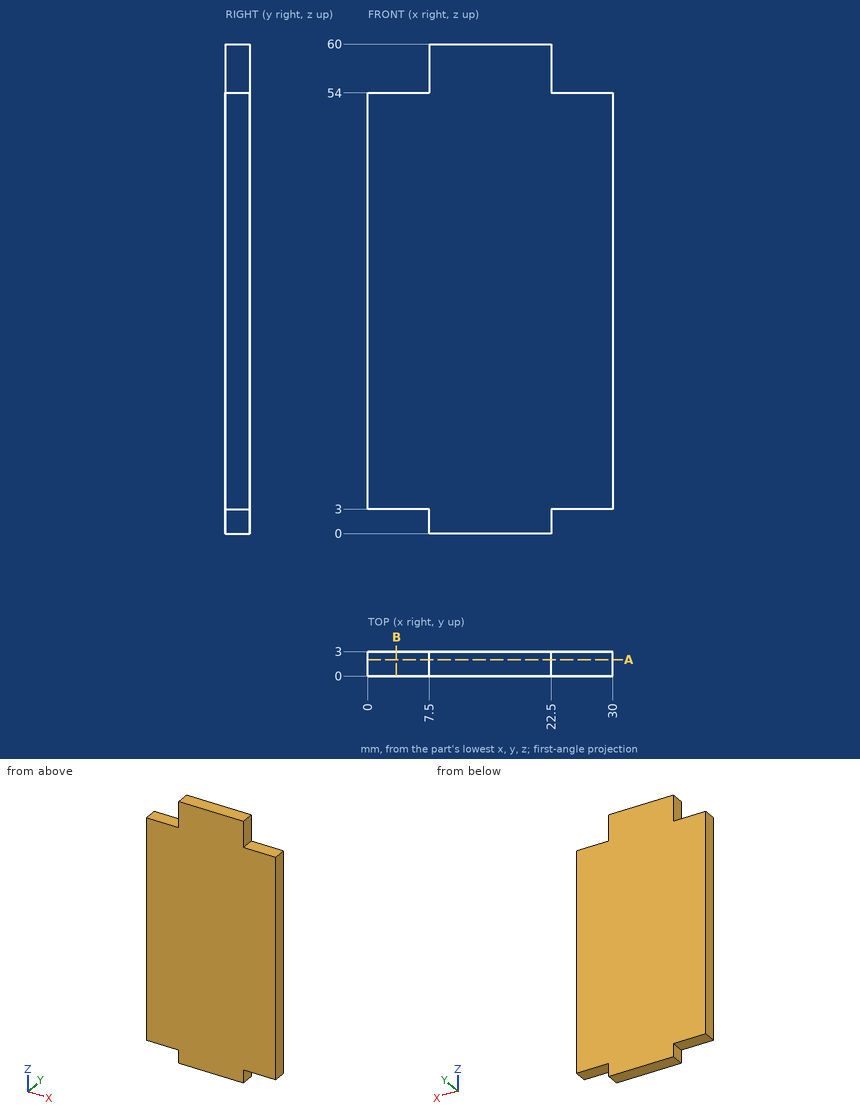
Job drawing, mm, ordinate dimensions from the low corner. One solid piece. Round coordinates to 2 decimals unless told otherwise and drop trailing zeros. Write each loop counter-clockwise with the first axis right and the second up, starting at its lowest first coordinate (ties: lowest second). Pieces come first, ordered by that corner, then holes. Notation, with made-up numbers: (87, 7) -> (124, 7) arc R30 ccw to (124, 42) -> close; hole circle Ø1 at (32, -13). An arc over 180 degrees is marked (long way). Answer as a JSON object with one key per item and string values.
(1) Probe probe 1 along X at (y, z) = (2.95, 55); probe 2 along Z at (x, y) = (27, 1.55). List the from-to ranges inside material, lowest first. Write a range as [from, to].
Reported:
{"probe 1": "x = [7.5, 22.5]", "probe 2": "z = [3, 54]"}
(2) Band-saw the part on A-A, the plane y = 2. List the corners of the cut face in (x, z), then the cut area to 4 significant figures.
Reported:
{"outline": "(0, 3) -> (7.5, 3) -> (7.5, 0) -> (22.5, 0) -> (22.5, 3) -> (30, 3) -> (30, 54) -> (22.5, 54) -> (22.5, 60) -> (7.5, 60) -> (7.5, 54) -> (0, 54) -> close", "area": "1,665 mm^2"}
(3) Band-saw the part on B-B, the plane x = 3.5. List the corners of the cut face in (y, z).
Reported:
{"outline": "(0, 3) -> (3, 3) -> (3, 54) -> (0, 54) -> close"}
(4) Pin check, flat tips, straight feed: P1, Ø1.5, axis at y = 1, z = 57, coming from the +X side; P2, Ø0.9, axis at x = 2, y = 1, coming from the -Z side; P3, Ø1.5, axis at x = 2.5, y = 1.5, coming from the +Z side. Stop position of each tip, or through.
Reported:
{"P1": "stops at x = 22.5", "P2": "stops at z = 3", "P3": "stops at z = 54"}
